Verification items for this drawing (mm, ordinates from the low corner). A direction names the side the tool comes from. Coordinates: 2 decimals unless noted, no trailing zeros. Write each loop counter-clockwise with the first axis right and the second up, starting at its lowest first coordinate (ties: lowest second). Pieces come first, ordered by that corner, then holes. Notation, with made-up numbers: (70.25, 49.5) -> (125.25, 49.5) arc R23 cw to (125.25, 58.5) -> close; hole circle Ø10 at (-24.5, -17). An arc over 180 degrees is marked (long way). Use CSV: the item, a comma, the result in double quotes.
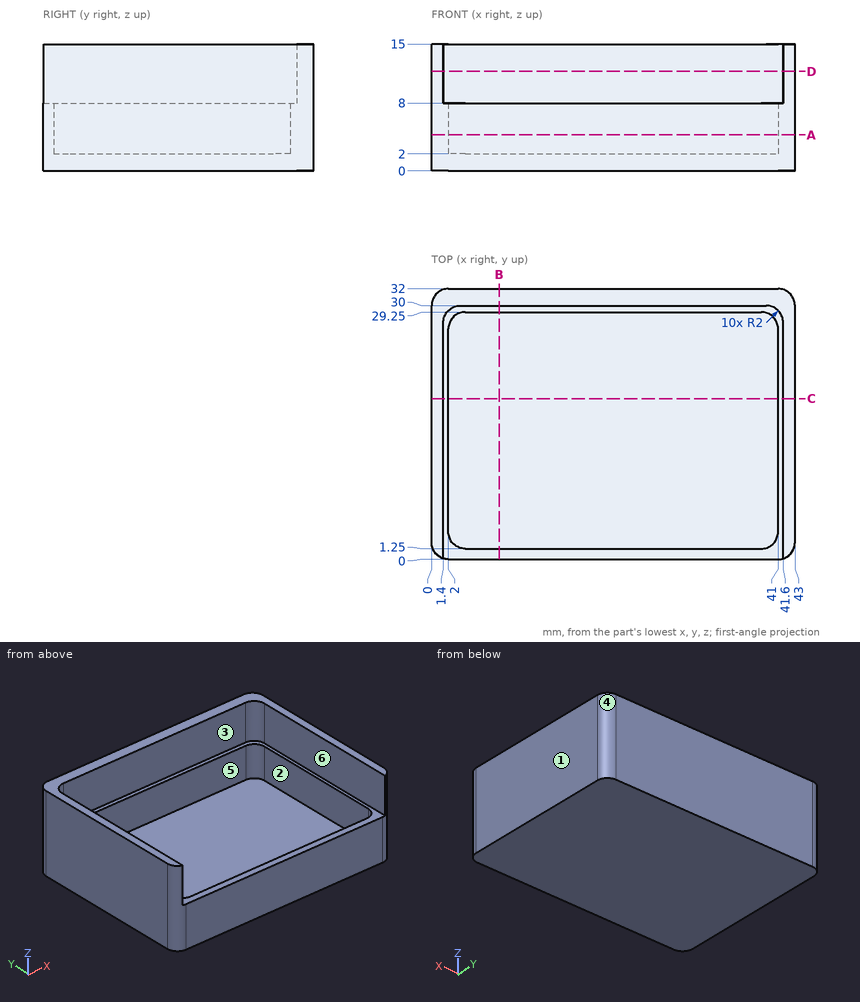
1) Set-up check for the marked faces 1, 2 and 3: record each of +Z, -Z, +X, -X, +Y, -Y from which the full face is reachable in a straight line by a thin tool's end or side.
Return value:
face 1,"+Z, -Z, +X, +Y, -Y"
face 2,"+Z"
face 3,"+Z, -Y"
2) Scan lines: L1, parallel to X at y = 15, z = 3.5; L2, parallel to X at y = 17, z = 10.25; L3, parallel to Y at x = 17, z = 3.75. Record each from-to range of solid material in increasing order.
Return value:
L1,"0 to 2, 41 to 43"
L2,"0 to 1.4, 41.6 to 43"
L3,"0 to 1.25, 29.25 to 32"
3) Cross-section at A-A (z = 4.25). Record the boundary of the cut face in (x, y), plus the area to 3 significant figures.
Return value:
outline,"(0, 2) arc R2 ccw to (2, 0) -> (41, 0) arc R2 ccw to (43, 2) -> (43, 30) arc R2 ccw to (41, 32) -> (2, 32) arc R2 ccw to (0, 30) -> close; hole (2, 3.25) arc R2 ccw to (4, 1.25) -> (39, 1.25) arc R2 ccw to (41, 3.25) -> (41, 27.25) arc R2 ccw to (39, 29.25) -> (4, 29.25) arc R2 ccw to (2, 27.25) -> close"
area,"284 mm2"
4) Cross-section at D-D (z = 11.75). Record the boundary of the cut face in (x, y), plus the area to 3 significant figures.
Return value:
outline,"(0, 2) arc R2 ccw to (1.4, 0.09) -> (1.4, 28) arc R2 cw to (3.4, 30) -> (39.6, 30) arc R2 cw to (41.6, 28) -> (41.6, 0.09) arc R2 ccw to (43, 2) -> (43, 30) arc R2 ccw to (41, 32) -> (2, 32) arc R2 ccw to (0, 30) -> close"
area,"168 mm2"
5) Cross-section at B-B (x = 8). Record the boundary of the cut face in (y, z), plus the area to 3 significant figures.
Return value:
outline,"(0, 0) -> (32, 0) -> (32, 15) -> (30, 15) -> (30, 8) -> (29.25, 8) -> (29.25, 2) -> (1.25, 2) -> (1.25, 8) -> (0, 8) -> close"
area,"102 mm2"
6) Cross-section at C-C (y = 19). Record the boundary of the cut face in (x, z).
Return value:
outline,"(0, 0) -> (43, 0) -> (43, 15) -> (41.6, 15) -> (41.6, 8) -> (41, 8) -> (41, 2) -> (2, 2) -> (2, 8) -> (1.4, 8) -> (1.4, 15) -> (0, 15) -> close"
7) Mould release check, pull along Y, two halves, no side actions. Record for the marked faces 4, 5 and 6: released by +Y, released by -Y, zero draft, split by the parting line, or undercut.
Return value:
face 4,"released by +Y"
face 5,"undercut"
face 6,"zero draft"
8) Gauge pin test, flat ends, axial feed: pin 1 (10 mm diameter, centred on x = 29.5, y = 9, fed in from +Z); pin 2 (3.5 mm diameter, centred on x = 22.5, z = 12, fed in from -Y). Record the tip position at first contact, or that the pin passes through.
Return value:
pin 1,"z = 2"
pin 2,"y = 30"
